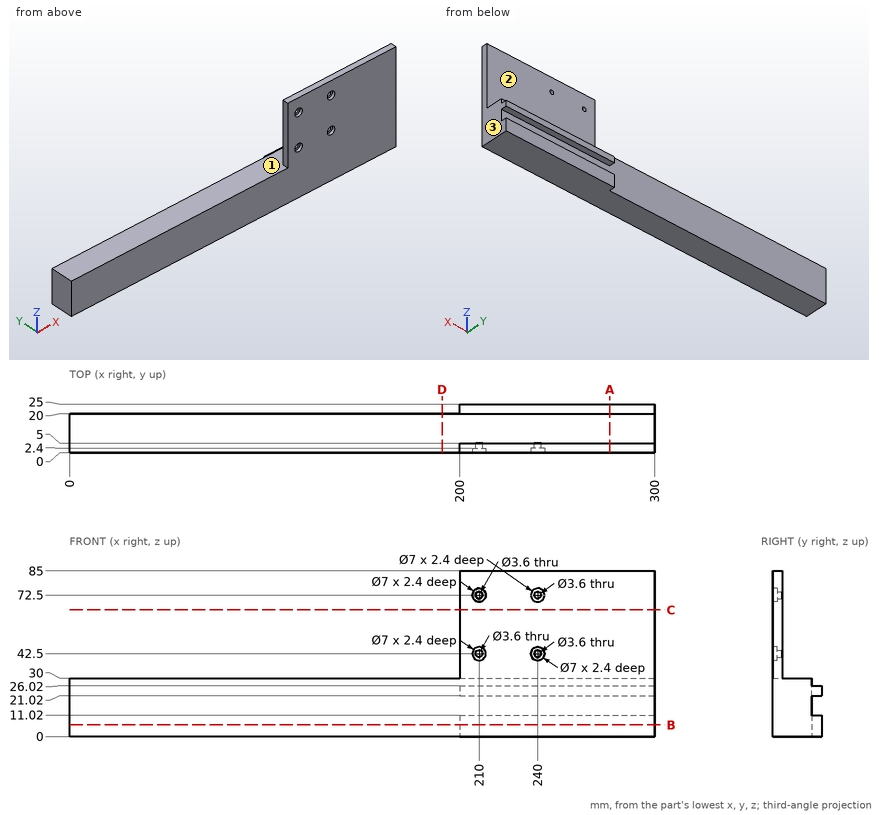
The drawing under review shows one solid part. Ordinate dimensions are in mm from its lowest x, y, z. A direction names the side the tool comes from. Coordinates: 2 decimals unless noted, no trailing zeros. Write each loop counter-clockwise with the first axis right and the second up, starting at its lowest first coordinate (ties: lowest second). Pieces come first, ordered by that corner, then holes. Notation, with made-up numbers: (39, 76.25) - (43, 76.25) arc R26 cw to (43, 95.25) - close; hole circle Ø9 at (29.25, 73). An arc over 180 degrees is marked (long way). Answer in a Markdown table with one row per item. Add a question column.
Q1. For probe 1 along Z at (x, y) = (240, 1.85); probe 2 along X at (y, z) = (1.7, 42.5); probe 3 along X at (y, z) = (3.45, 42.5), list the stretches that pass through material, from the lowest coordinate up.
Q2. We need section D-D, the plane x = 191. State the section outline as (y, z) points.
Q3. We need section C-C, the plane z = 65. State the section outline as (x, y) points.
Q4. We need section B-B, the plane z = 6. State the section outline as (x, y) points, and give its area (3 significant figures).
Q5. We need section A-A, the plane x = 277. State the section outline as (y, z) points.
Q6. Tool access review of the marked faces 1, 2 and 3: name each direction out of +Z, -Z, +X, -X, +Y, -Y from which nothing blocks a thin tool from reaching the whole face with its end or side.
Q7. For P1, Ø4.5, axis at x = 210, z = 42.5, coming from the +Y side; P2, Ø1, axis at x = 207.5, y = 11.5, coming from the -Z side; P3, Ø4, axis at x = 257.5, y = 23.5, coming from the +Z side; P4, Ø1.5, axis at y = 22, z = 24, coming from the -X side, all flat-tipped, find the tip position at first contact; note any pin that passes through.
Answer list:
| question | item | result |
|---|---|---|
| 1 | probe 1 | z = 0 to 39, 46 to 69, 76 to 85 |
| 1 | probe 2 | x = 200 to 206.5, 213.5 to 236.5, 243.5 to 300 |
| 1 | probe 3 | x = 200 to 208.2, 211.8 to 238.2, 241.8 to 300 |
| 2 | outline | (0, 0) - (20, 0) - (20, 30) - (0, 30) - close |
| 3 | outline | (200, 0) - (300, 0) - (300, 5) - (200, 5) - close |
| 4 | outline | (0, 0) - (300, 0) - (300, 25) - (200, 25) - (200, 20) - (0, 20) - close |
| 4 | area | 6,500 mm2 |
| 5 | outline | (0, 0) - (25, 0) - (25, 11.02) - (20, 11.02) - (20, 21.02) - (25, 21.02) - (25, 26.02) - (20, 26.02) - (20, 30) - (5, 30) - (5, 85) - (0, 85) - close |
| 6 | face 1 | +Z, -X, +Y |
| 6 | face 2 | +Z, +X, -X, +Y |
| 6 | face 3 | +Z, -Z, +X, +Y, -Y |
| 7 | P1 | stops at y = 5 |
| 7 | P2 | stops at z = 0 |
| 7 | P3 | stops at z = 26.02 |
| 7 | P4 | stops at x = 200 |
